from build123d import *

# Parameters (mm, degrees)
EXTRUDE_THIN1_DEPTH      = 215.9
EXTRUDE_THIN1_DEPTH_BACK = 203.2
SKETCH2_R                = 6.35
CUT_EXTRUDE1_DEPTH       = 7.35


with BuildPart() as part:
    # Sketch1 → Extrude-Thin1 (new body, two sides)
    with BuildSketch(Plane.XY) as extrude_thin1_sk:
        Polygon((-269.875, 946.3), (-269.875, 984.4), (-307.975, 984.4), (-307.975, 978.05), (-276.225, 978.05), (-276.225, 946.3), align=None)
    extrude(amount=EXTRUDE_THIN1_DEPTH)
    extrude(extrude_thin1_sk.sketch, amount=-EXTRUDE_THIN1_DEPTH_BACK)

    # Sketch2 → Cut-Extrude1 (cut, through all)
    with BuildSketch(Plane.ZY.offset(276.225)):
        with Locations((109.908874461, 962.175)):
            Circle(SKETCH2_R)
        with Locations((71.808874461, 962.175)):
            Circle(SKETCH2_R)
    extrude(amount=-CUT_EXTRUDE1_DEPTH, mode=Mode.SUBTRACT)


solid = part.part
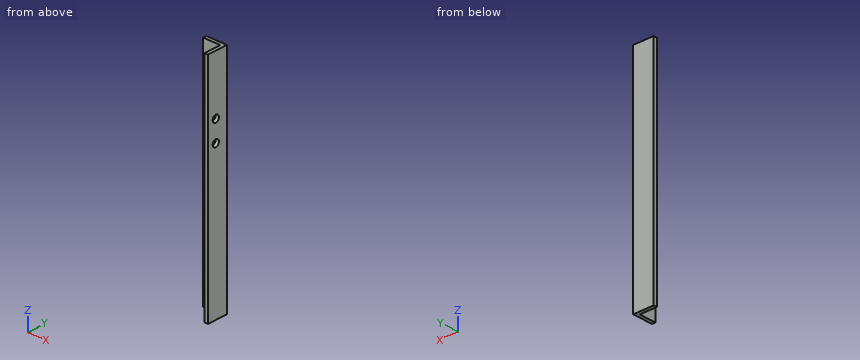
Input: part model. Units: mm. Frame: model coordinates. Give positions to 0.01 mm unless a question says otherwise; leave off trailing zeros. Write each loop counter-clockwise with the first axis right and the second up, starting at its lowest first coordinate (ties: lowest second). Pieces come first, ordered by that corner, then holes. Notation, with made-up numbers: M -14.5,4 L 10.5,4 A28 cw 10.5,23 Z; hole C -35.75,81.5 d10. An arc over 180 degrees is marked long. Write item = value, one per line. Start each with the question number.
1) Cut plane D-D on x = -297.5. Return the cut outline in (y, z), then the cut area to 3 significant figures.
2) First-contact query: pin 1 Ø7.5 at (y, z) = (962.18, 109.91) entering from +X; pin 2 Ø10 at (x, z) = (-291, -115) entering from -Y. Flat tips, straight axial feed; report the tip coordinate or a pass-through.
3) Cut plane B-B on z = 12. Return the cut outline in (x, y) (3 decimals).
4) Material intervals for line 1 along X through (y, z) = (967, 38) (3 decimals); line 2 along Y through (x, z) = (-284, -65); line 3 along Z through (x, y) = (-274.5, 959), sorted ascending. Write a range as [from, to].
5) Cut plane C-C on y = 950. Return the cut outline in (x, z) (3 decimals), then the cut area to 3 significant figures.
6) Cut plane A-A on z = 73. Return the cut outline in (x, y) (3 decimals).
Solved:
q1.outline = M 978.05,-203.2 L 984.4,-203.2 L 984.4,215.9 L 978.05,215.9 Z
q1.area = 2,660 mm2
q2.pin_1 = through
q2.pin_2 = 978.05
q3.outline = M -307.975,978.05 L -276.225,978.05 L -276.225,946.3 L -269.875,946.3 L -269.875,984.4 L -307.975,984.4 Z
q4.line_1 = [-276.225, -269.875]
q4.line_2 = [978.05, 984.4]
q4.line_3 = [-203.2, 66.31], [77.31, 104.41], [115.41, 215.9]
q5.outline = M -276.225,-203.2 L -269.875,-203.2 L -269.875,215.9 L -276.225,215.9 Z
q5.area = 2,660 mm2
q6.outline = M -307.975,978.05 L -276.225,978.05 L -276.225,968.412 L -269.875,968.412 L -269.875,984.4 L -307.975,984.4 Z; M -276.225,946.3 L -269.875,946.3 L -269.875,955.938 L -276.225,955.938 Z
